Answer from the drawing. Dimensions are ordinates in mm from the lowest x, y and z of the part. A direction names the side the tool comes from. Round coordinates to 2 decimals unless told otherwise and drop trailing zeros. Write each loop counter-clockwise with the first axis right and the second up, starting at its lowest first coordinate (ties: lowest second). Pieces come first, ordered by that corner, then holes. Notation, with made-up numbers: (56.5, 40) -> (85.5, 40) arc R13 ccw to (85.5, 58) -> close; hole circle Ø4 at (-33.75, -12). An arc over 180 degrees is marked (long way). Return JSON: item names as keys, results as strings. Group by question number.
(1) A cutting plane is placed at D-D on y = 17.25. Give the vertices of the cut face in (x, z).
(2) A cutting plane is placed at A-A on x = 14. Give the vertices of the cut face in (y, z), then the cut area to 3 significant figures.
(3) The mould has two halves that part along X. Classify the marked faces 1, 2 and 3: released by +X, released by -X, zero draft, split by the parting line, or undercut.
(4) Given pin 1 (1.5 mm diameter, centred on y = 10.5, z = 4, fed in from -X); pin 2 (8 mm diameter, centred on y = 6.5, z = 16.5, fed in from +X); pin 3 (5 mm diameter, centred on x = 4, y = 3.5, fed in from -Z); pin 4 (12 mm diameter, centred on y = 13.5, z = 19, fed in from -X), each flat-ended and moving along its own axis, determine where each tip first touches the part or whether it passes through.
(5) A cutting plane is placed at B-B on z = 14. Give the vertices of the cut face in (x, y).
(6) Straight lines are drawn through the part: line 1 (Z direction, x = 14.25, y = 10.75); line 2 (Y direction, x = 23, z = 19); line 3 (Z direction, x = 15, y = 19.75). For each, find the intervals that lie inside material, in ascending order.
(7) For the marked faces 4 and 5, determine the directions among +Z, -Z, +X, -X, +Y, -Y from which every point of the face is accessible in a straight line to the end or side of a thin tool.
(8) A cutting plane is placed at C-C on z = 20. Give the vertices of the cut face in (x, y), then the cut area to 3 significant figures.
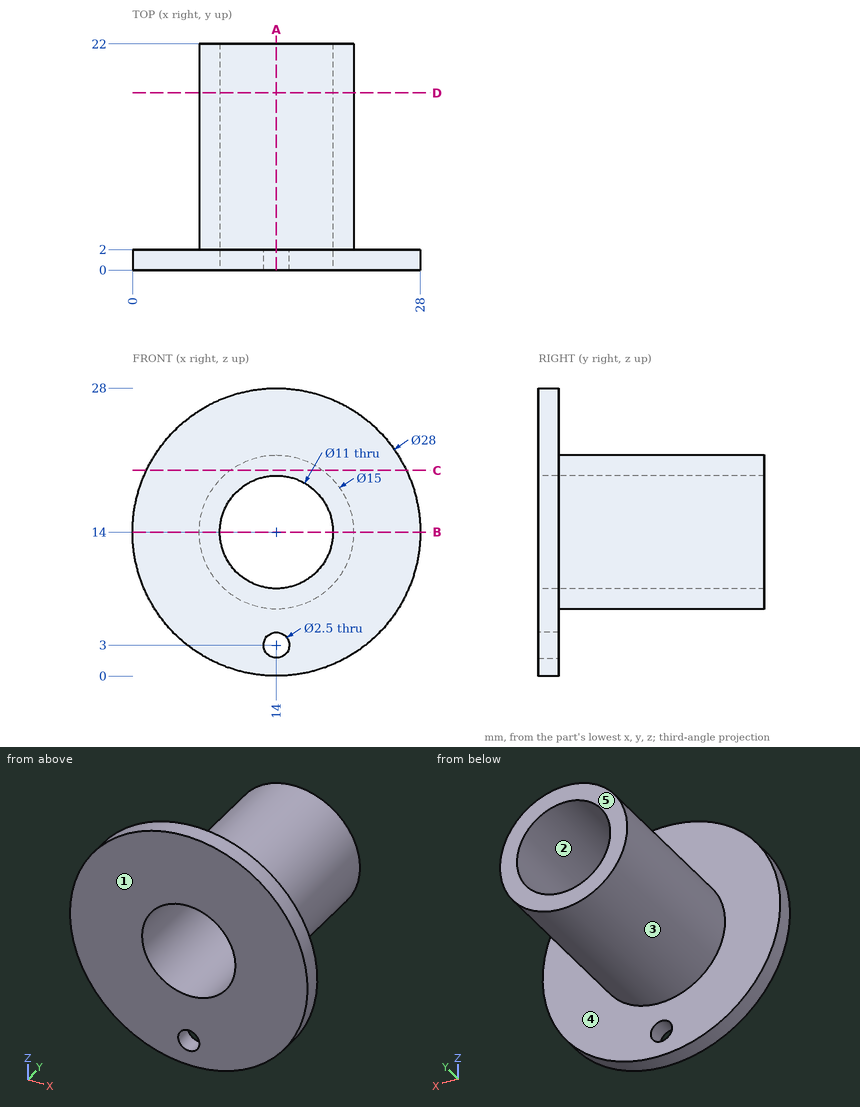
Checks:
{
 "1": {"outline": "circle Ø15 at (14, 14); hole circle Ø11 at (14, 14)"},
 "2": {"outline": "(0, 0) -> (2, 0) -> (2, 1.75) -> (0, 1.75) -> close; (0, 4.25) -> (2, 4.25) -> (2, 6.5) -> (22, 6.5) -> (22, 8.5) -> (0, 8.5) -> close; (0, 19.5) -> (22, 19.5) -> (22, 21.5) -> (2, 21.5) -> (2, 28) -> (0, 28) -> close", "area": "109 mm^2"},
 "3": {"face 1": "zero draft", "face 2": "undercut", "face 3": "split by the parting line"},
 "4": {"pin 1": "passes through", "pin 2": "stops at x = 21.5", "pin 3": "stops at z = 2.51", "pin 4": "stops at x = 6.5"},
 "5": {"outline": "(0, 0) -> (8.5, 0) -> (8.5, 22) -> (6.5, 22) -> (6.5, 2) -> (0, 2) -> close; (19.5, 0) -> (28, 0) -> (28, 2) -> (21.5, 2) -> (21.5, 22) -> (19.5, 22) -> close"},
 "6": {"line 1": "z = 6.5 to 8.51, 19.49 to 21.5", "line 2": "y = 0 to 2", "line 3": "z = 6.57 to 8.59, 19.41 to 21.43"},
 "7": {"face 4": "+Y", "face 5": "+Z, -Z, +X, -X, +Y"},
 "8": {"outline": "(1.35, 0) -> (26.65, 0) -> (26.65, 2) -> (18.5, 2) -> (18.5, 22) -> (9.5, 22) -> (9.5, 2) -> (1.35, 2) -> close", "area": "231 mm^2"}
}
